from build123d import *

# Parameters (mm, degrees)
F0_R           = 1.7
F1_DEPTH       = 2
F2_R           = 5
F3_D           = 3
F3_DEPTH       = 13.5
F3_CSINK_D     = 5.4
F3_CSINK_ANGLE = 75
F4_DEPTH       = 25
F5_R           = 1


with BuildPart() as f1:
    # F0 (on Front) → F1 (new body)
    with BuildSketch(Plane.XZ):
        with BuildLine():
            Line((0, 38), (-88, 38))
            Line((-88, 38), (-88, 0))
            Line((-88, 0), (-26.377132, 0))
            Line((-26.377132, 0), (-26.377132, 5.6))
            ThreePointArc((-26.377132, 5.6), (-24.613067, 7.364066), (-22.849001, 5.6))
            Line((-22.849001, 5.6), (-22.849001, 0))
            Line((-22.849001, 0), (0, 0))
            Line((0, 0), (0, 38))
        make_face()
        with Locations((-84.8, 4.8)):
            Circle(F0_R, mode=Mode.SUBTRACT)
        with Locations((-3.2, 4.8)):
            Circle(F0_R, mode=Mode.SUBTRACT)
        with Locations((-84.8, 33.2)):
            Circle(F0_R, mode=Mode.SUBTRACT)
        with Locations((-3.2, 33.2)):
            Circle(F0_R, mode=Mode.SUBTRACT)
        with BuildLine():
            Line((-26.377132, 5.6), (-26.377132, 0))
            Line((-26.377132, 0), (-22.849001, 0))
            Line((-22.849001, 0), (-22.849001, 5.6))
            ThreePointArc((-22.849001, 5.6), (-24.613067, 7.364066), (-26.377132, 5.6))
        make_face()
    extrude(amount=-F1_DEPTH)

    # F2
    f2_edges = [f1.edges().sort_by_distance(p)[0] for p in [
        (-88, 1, 38),
        (-88, 1, 0),
        (0, 1, 0),
        (0, 1, 38),
    ]]
    fillet(f2_edges, radius=F2_R)

    # F3
    with Locations(Plane.XZ):
        with Locations((-84.8, 4.8), (-84.8, 33.2), (-3.2, 4.8), (-3.2, 33.2)):
            CounterSinkHole(F3_D / 2, F3_CSINK_D / 2, depth=F3_DEPTH, counter_sink_angle=F3_CSINK_ANGLE)

    # F0 (on Front) → F4 (cut)
    with BuildSketch(Plane.XZ):
        with BuildLine():
            Line((-26.377132, 5.6), (-26.377132, 0))
            Line((-26.377132, 0), (-22.849001, 0))
            Line((-22.849001, 0), (-22.849001, 5.6))
            ThreePointArc((-22.849001, 5.6), (-24.613067, 7.364066), (-26.377132, 5.6))
        make_face()
    extrude(amount=-F4_DEPTH, mode=Mode.SUBTRACT)

    # F5
    f5_edges = [f1.edges().sort_by_distance(p)[0] for p in [
        (-26.377132, 1, 0),
        (-22.849001, 1, 0),
    ]]
    fillet(f5_edges, radius=F5_R)


solid = f1.part
Source: CAD feature listing. Evaluate the final solid. Frame: model axes, mm. A direction names the side the tool comes from. Coordinates: 2 decimals unless noted, no trailing zeros. Loops run counter-clockwise (first coordinate to the right, second up) from the corner with the lowest first, then second, coordinate; pieces in that order, holes last. Notation, with made-up numbers: (27, -39) -> (58, -39) arc R16 cw to (58, -33) -> close; hole circle Ø6 at (53, -26). An arc over 180 degrees is marked (long way). Answer in a Markdown table with one row per item. Add a question column.
Q1. Ray query, line 1 along X through (y, z) = (1.8, 4.8); line 2 along X through (y, z) = (1.7, 33.2); line 3 along X through (y, z) = (0.8, 36). Return the intervals inside material, ascending.
Q2. Section C-C on z = 34. Give the number of separate pieces and of enclosed holes in the cut face, and give its area (3 significant figures).
Q3. Reachability of faces 1 (the face through (-45, 0, 19)), 2 (the face through (-22.849, 1, 3)) from +Z, -Z, +X, -X, +Y, -Y: full face, straight path, thin tool, end or side. Return the list, or none.
Q4. Contact query for a flat-ended pin moving along its axis: pin 1 Ø4 at (x, z) = (-84.8, 4.8) entering from +Y. Output: stop coordinate, or through.
Q5. Pull-direction query (X, two-part tool) for faces 3 (the face through (-4.9, 1.65, 4.87)), 4 (the face through (-83.18, 1.65, 33.71)), 5 (the face through (-88, 1, 19)), 6 (the face through (-45, 2, 19)); classes: pulls with the +X half, pulls with the -X half, needs draft (parallel to the pull), parting line crosses it, or undercut.
Q6. Section B-B on x = -3.2. Return the cut outline in (y, z), and give its area (3 significant figures).
Q7. Section D-D on x = -24.5. Return the cut outline in (y, z).
Q8. Section A-A on y = 1.7. Return the cut outline in (x, z).
Computed values:
| question | item | result |
|---|---|---|
| 1 | line 1 | x = -88 to -86.5, -83.1 to -26.38, -22.85 to -4.9, -1.5 to 0 |
| 1 | line 2 | x = -88 to -86.5, -83.1 to -4.9, -1.5 to 0 |
| 1 | line 3 | x = -87 to -1 |
| 2 | separate pieces | 3 |
| 2 | enclosed holes | 0 |
| 2 | area | 161 mm^2 |
| 3 | face 1 | +Z, -Z, +X, -X, -Y |
| 3 | face 2 | -Z, +Y, -Y |
| 4 | pin 1 | stops at y = 2 |
| 5 | face 3 | undercut |
| 5 | face 4 | undercut |
| 5 | face 5 | pulls with the -X half |
| 5 | face 6 | needs draft |
| 6 | outline | (0, 0.34) -> (2, 0.34) -> (2, 3.1) -> (1.3, 3.1) -> (0, 2.1) -> close; (0, 7.5) -> (1.3, 6.5) -> (2, 6.5) -> (2, 31.5) -> (1.3, 31.5) -> (0, 30.5) -> close; (0, 35.9) -> (1.3, 34.9) -> (2, 34.9) -> (2, 37.66) -> (0, 37.66) -> close |
| 6 | area | 58.5 mm^2 |
| 7 | outline | (0, 7.36) -> (2, 7.36) -> (2, 38) -> (0, 38) -> close |
| 8 | outline | (-88, 5) arc R5 ccw to (-83, 0) -> (-27.38, 0) arc R1 ccw to (-26.38, 1) -> (-26.38, 5.6) arc R1.76 cw to (-22.85, 5.6) -> (-22.85, 1) arc R1 ccw to (-21.85, 0) -> (-5, 0) arc R5 ccw to (0, 5) -> (0, 33) arc R5 ccw to (-5, 38) -> (-83, 38) arc R5 ccw to (-88, 33) -> close; hole circle Ø3.4 at (-84.8, 4.8); hole circle Ø3.4 at (-84.8, 33.2); hole circle Ø3.4 at (-3.2, 4.8); hole circle Ø3.4 at (-3.2, 33.2) |
